from build123d import *

# Parameters (mm, degrees)
SKETCH_2_R      = 4
EXTRUDE_1_DEPTH = 21.5
EXTRUDE_2_DEPTH = 6
CHAMFER_1_SIZE  = 1


with BuildPart() as part:
    # 草圖2 → 伸長1 (new body)
    with BuildSketch(Plane.XY):
        Circle(SKETCH_2_R)
    extrude(amount=EXTRUDE_1_DEPTH)

    # 草圖3 → 伸長2 (add)
    with BuildSketch(Plane(origin=(0, 0, 0), x_dir=(-1, 0, 0), z_dir=(0, 0, -1))):
        Polygon((3.464101615, -6), (6.92820323, 0), (3.464101615, 6), (-3.464101615, 6), (-6.92820323, 0), (-3.464101615, -6), align=None)
    extrude(amount=EXTRUDE_2_DEPTH)

    # 草圖5 → 除料-旋轉1 (revolve, cut)
    with BuildSketch(Plane(origin=(0, 0, 0), x_dir=(1, 0, 0), z_dir=(0, 1, 0)), mode=Mode.PRIVATE) as cut_revolve_1_sk:
        Polygon((6.92820323, 5.464101615), (6.92820323, 6), (6, 6), align=None)
    revolve(cut_revolve_1_sk.sketch.rotate(Axis((0, 0, 0), (0, 0, -1)), 180), axis=Axis((0, 0, 0), (0, 0, -1)), mode=Mode.SUBTRACT)

    # 導角1
    chamfer_1_edges = [part.edges().sort_by_distance(p)[0] for p in [
        (-4, 0, 21.5),
    ]]
    chamfer(chamfer_1_edges, length=CHAMFER_1_SIZE)


solid = part.part
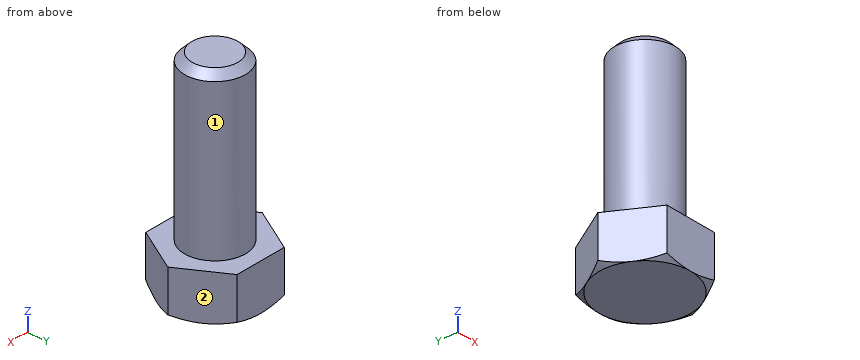
Here's how the part is built. I have some questions about the finished solid (model axes, mm). Face numbers are marked on the shaded views. A direction names the side the tool comes from. Round coordinates to 2 decimals unless told otherwise and drop trailing zeros. Order: outer loops, then holes, each group sorted by start corner. A loop starts at its lowest first (then second) coordinate and runs counter-clockwise, first axis right, second up. Notation, with made-up numbers: (-4.5, 1.25) -> (24.5, 1.25) arc R33 cw to (24.5, 32.25) -> close; hole circle Ø3 at (19.5, 13.25). An arc over 180 degrees is marked (long way). Return JSON: item names as keys, results as strings.
Q1. If we section it at A-A on z = -2: List the corners of the cut face in (x, y) for me.
Filled sheet:
{"outline": "(-6.93, 0) -> (-3.46, -6) -> (3.46, -6) -> (6.93, 0) -> (3.46, 6) -> (-3.46, 6) -> close"}
Q2. Which directions (+Z, -Z, +X, -X, +Y, -Y) give clear straight access to the entire face, cutting with the end or side of a thin tool? Please do the marked faces 1 and 2.
Filled sheet:
{"face 1": "+Z", "face 2": "+Z, -Z, +X, +Y"}
Q3. If we section it at B-B on z = 2.5: List the corners of the cut face in (x, y) for me.
Filled sheet:
{"outline": "circle Ø8 at (0, 0)"}
Q4. For pin 1 Ø1 at (x, y) = (-2, 4.5) entering from +Z; pin 2 Ø1 at (x, z) = (5.5, -1) entering from +Y; pin 3 Ø1 at (x, z) = (1.5, 12.5) entering from -Y, each with a flat end and sliding along its axis, tell me the tip position at first contact or that it passes through.
Filled sheet:
{"pin 1": "stops at z = 0", "pin 2": "stops at y = 3.34", "pin 3": "stops at y = -3.87"}
Q5. I need wall thicknesses on line 1 along Z through (x, y) = (4.25, 2.5); line 2 along Z through (x, y) = (-3.25, 2); line 3 along Y through (x, z) = (2.5, 4.25). Which ranges of each line are inside material? Lowest first, please. Write a range as from..to.
Filled sheet:
{"line 1": "z = -6..0", "line 2": "z = -6..20.68", "line 3": "y = -3.12..3.12"}
